Source: CAD feature listing. Evaluate the final solid. Frame: model axes, mm. Give positions to 0.01 mm unless a question says otherwise; leave off trailing zeros. Answer as a JSON object with one key per item and string values. Group by question number.
from build123d import *

# Parameters (mm, degrees)
EXTRUDE_1_DEPTH          = 0.5
PATTERN_CIRCULAR_1_COUNT = 2


with BuildPart() as part:
    # 草图1 → 凸台-拉伸1 (new body)
    with BuildSketch(Plane(origin=(0, 0, 0), x_dir=(1, 0, 0), z_dir=(0, 1, 0))):
        with BuildLine():
            Line((-11.5, 0), (11.5, 0))
            ThreePointArc((11.5, 0), (12.207106781, 0.292893219), (12.5, 1))
            Line((12.5, 1), (12.5, 24))
            ThreePointArc((12.5, 24), (12.207106781, 24.707106781), (11.5, 25))
            Line((11.5, 25), (-11.5, 25))
            ThreePointArc((-11.5, 25), (-12.207106781, 24.707106781), (-12.5, 24))
            Line((-12.5, 24), (-12.5, 1))
            ThreePointArc((-12.5, 1), (-12.207106781, 0.292893219), (-11.5, 0))
        make_face()
    extrude(amount=EXTRUDE_1_DEPTH)


with BuildPart() as pattern_circular_1_1:
    # 阵列(圆周)1: pattern copy
    add(part.part.rotate(Axis((0, 0, 0), (0, 1, 0)), 1 * 360 / PATTERN_CIRCULAR_1_COUNT))


with BuildPart() as part_1:
    add(part.part)

    # Combine 1: union 阵列(圆周)1_1
    add(pattern_circular_1_1.part)


solid = part_1.part
Q1. Ray query, probe 1 along X at (y, z) = (0.2, -0.5). Return the intervals inside material, ascending. Write a range as [from, to].
Q2. First-contact query: pin 1 Ø6 at (x, z) = (5.5, 14.5) entering from -Y. Flat tip, straight axial feed; report the tip coordinate or a pass-through.
Q3. Draft query along Z for faces 1 (the cylindrical face through (12.199, 0.246, 24.715)), 2 (the cylindrical face through (-12.199, 0.246, 0.285)), 3 (the flat face through (0, 0, 0)). Return one class per face: released by +Z, released by -Z, zero draft, split by the parting line, or undercut.
Taken from the geometry:
{
 "1": {"probe 1": "x = [-12.37, 12.37]"},
 "2": {"pin 1": "stops at y = 0"},
 "3": {"face 1": "released by +Z", "face 2": "undercut", "face 3": "zero draft"}
}
